Check sheet for the modelled part. Datum: model origin and axes. Units: mm. A direction names the side the tool comes from. Round coordinates to 2 decimals unless told otherwise and drop trailing zeros. Order: outer loops, then holes, each group sorted by start corner. A loop starts at its lowest first (then second) coordinate and runs counter-clockwise, first axis right, second up.
```python
from build123d import *

# Parameters (mm, degrees)
F1_DEPTH = 63.5
F2_DEPTH = 25.4
F3_DEPTH = 7.9375
F5_R     = 12.877415


with BuildPart() as f1:
    # F0 (on Front) → F1 (new body, symmetric)
    with BuildSketch(Plane.XZ):
        Polygon((22.86, 9.525), (-41.275, 9.525), (-41.275, -9.525), (41.275, -9.525), (41.275, 9.525), align=None)
    extrude(amount=F1_DEPTH, both=True)

    # F0 (on Front) → F2 (join, symmetric)
    with BuildSketch(Plane.XZ):
        with BuildLine():
            Line((22.86, 27.554785), (22.86, 9.525))
            Line((22.86, 9.525), (41.275, 9.525))
            Line((41.275, 9.525), (41.275, 27.554785))
            ThreePointArc((41.275, 27.554785), (47.109768, 39.851507), (60.325, 43.109045))
            Line((60.325, 43.109045), (60.325, 61.486875))
            add(Edge.make_bspline(
                [(54.669271, 61.754933), (56.556617, 61.689986), (58.442735, 61.599782), (60.325, 61.486875)],
                knots=[108.732471, 108.732471, 108.732471, 108.732471, 113.939403, 113.939403, 113.939403, 113.939403], degree=3))
            ThreePointArc((54.669271, 61.754933), (32.041552, 50.907942), (22.86, 27.554785))
        make_face()
        with BuildLine():
            Line((60.325, 66.675), (60.325, 61.697478))
            ThreePointArc((60.325, 61.697478), (61.813019, 61.526249), (63.29214, 61.2902))
            add(Edge.make_bspline(
                [(60.325, 61.486875), (61.31524, 61.427476), (62.304414, 61.361794), (63.29214, 61.2902)],
                knots=[113.939403, 113.939403, 113.939403, 113.939403, 116.678715, 116.678715, 116.678715, 116.678715], degree=3))
            Line((60.325, 61.486875), (60.325, 43.109045))
            ThreePointArc((60.325, 43.109045), (60.819058, 42.999967), (61.309388, 42.8752))
            Line((61.309388, 42.8752), (85.725, 42.8752))
            Line((85.725, 42.8752), (85.725, 66.675))
            Line((85.725, 66.675), (60.325, 66.675))
        make_face()
    extrude(amount=F2_DEPTH, both=True)

    # F0 (on Front) → F3 (join, symmetric)
    with BuildSketch(Plane.XZ):
        with BuildLine():
            add(Edge.make_bspline(
                [(-41.275, 9.525), (-24.690354, 53.453726), (15.257235, 63.111172), (54.669271, 61.754933)],
                knots=[0, 0, 0, 0, 108.732471, 108.732471, 108.732471, 108.732471], degree=3))
            Line((-41.275, 9.525), (22.86, 9.525))
            Line((22.86, 9.525), (22.86, 27.554785))
            ThreePointArc((22.86, 27.554785), (32.041552, 50.907942), (54.669271, 61.754933))
        make_face()
    extrude(amount=F3_DEPTH, both=True)

    # F0 (on Front) → F4 (revolve)
    with BuildSketch(Plane.XZ):
        Polygon((111.125, 66.675), (85.725, 66.675), (85.725, 42.8752), (85.725, 38.1), (111.125, 38.1), align=None)
    revolve(axis=Axis((85.725, 0, 52.3875), (0, 0, -1)))

    # F5
    f5_edges = [f1.edges().sort_by_distance(p)[0] for p in [
        (41.275, -63.5, 0),
        (-41.275, -63.5, 0),
        (-41.275, 63.5, 0),
        (41.275, 63.5, 0),
    ]]
    fillet(f5_edges, radius=F5_R)


solid = f1.part
```
Item 1: Scan lines: line 1 along Y through (x, z) = (74.5, 59.5); line 2 along Z through (x, y) = (-10.5, 27.5) (3 decimals); line 3 along X through (y, z) = (12, 3) (3 decimals). Record each from-to range of solid material in increasing order.
Answer:
line 1: y = -25.4 to 25.4
line 2: z = -9.525 to 9.525
line 3: x = -41.275 to 41.275
Item 2: Go/stop test with flat-tipped pins: P1, Ø14, axis at y = -20, z = 19, coming from the -X side; P2, Ø12, axis at x = 44.5, z = 4.5, coming from the -Y side; P3, Ø20, axis at x = 70, y = 17.5, coming from the -Z side. Record where each tip stops, or that it passes through.
Answer:
P1: stops at x = 22.86
P2: stops at y = -58.61
P3: stops at z = 38.1
Item 3: Sectioned sample at A-A (z = -3). Record the cut outline in (x, y) (3 decimals).
Answer:
outline: (-41.275, -50.623) arc R12.877 ccw to (-28.398, -63.5) - (28.398, -63.5) arc R12.877 ccw to (41.275, -50.623) - (41.275, 50.623) arc R12.877 ccw to (28.398, 63.5) - (-28.398, 63.5) arc R12.877 ccw to (-41.275, 50.623) - close
Item 4: Release check for a two-part mould opening along Y. For faces 4 (the cylindrical face through (109.95, -7.63, 49.41)), 5 (the flat face through (85, 0, 66.675)), 6 (the flat face through (54, 25.4, 45)), 7 (the cylindrical face through (37.4, -59.83, 0.13)) record: released by +Y, released by -Y, zero draft, split by the parting line, or undercut.
Answer:
face 4: split by the parting line
face 5: zero draft
face 6: released by +Y
face 7: released by -Y
Item 5: Access from +Z, -Z, +X, -X, +Y, -Y to the whole of each face (thin tool, end or side, straight path). Record for faces 1 (the flat face through (54, -25.4, 45)), 2 (the cylindrical face through (32.29, 16.55, 51.17)), 3 (the flat face through (22.86, -17, 19)).
Answer:
face 1: +Z, +X, -X, -Y
face 2: +Z, -X, +Y
face 3: +Z, -X, -Y
